CAD build for the part. Positions are in the model's coordinates, mm. A direction names the side the tool comes from. Coordinates: 2 decimals unless noted, no trailing zeros. Write each loop counter-clockwise with the first axis right and the second up, starting at its lowest first coordinate (ties: lowest second). Pieces come first, ordered by that corner, then holes. Notation, with made-up numbers: (39, 25.25) - (93, 25.25) arc R16 cw to (93, 37.25) - close; hole circle Ø8 at (-7.75, 73). An arc over 180 degrees is marked (long way). One line per question, with ' | ' between items. Start each with the question number.
1. Band-saw the part on A-A, the plane x = 0. Write the cut outline in (y, z).
2. Probe line 1 (Z direction, x = -55, y = -20); line 2 (X direction, y = 0, z = -2.25); line 3 (Y direction, x = 0, z = 5.75). List the from-to ranges inside material, lowest first.
3. Two-plate mould, pull along Z, no slides. Class faces 1 (the flat face through (-1, 13, -6.35)), 2 (the flat face through (-1, -13, 12.7)), 3 (the cylindrical face through (-43.06, 39.48, 3.13)), 4 (the flat face through (-10, 58, 6.35)): +Z half, -Z half, draft (parallel to the pull), parting line (faces both ways), or undercut.
4. Band-saw the part on D-D, the plane z = 9.5. Write the cut outline in (x, y), then the cut area to 3 significant figures.
5. Band-saw the part on C-C, the plane x = 23. Write the cut outline in (y, z).
6. Flat gauge pins, fed straight in: P1, Ø8, axis at x = -25, z = 3, coming from the -Y side; P2, Ø3, axis at y = -3.5, z = 2, coming from the -X side; P3, Ø1, axis at y = 2, z = 3, coming from the +X side. Where does each tip first touch, or does it go through?
7. Which spindle directions (+Z, -Z, +X, -X, +Y, -Y) get a long thin tool onto all of the face, cutting with end or side? Do faces 5 (the cylindrical face through (-0.83, 3.72, 3.31)), 6 (the flat face through (-10, -58, 0)). Say none if no direction does.
from build123d import *

# Parameters (mm, degrees)
F0_R     = 58.42
F1_DEPTH = 6.35
F2_R     = 3.81
F3_DEPTH = 25.4
F4_R     = 64.77
F4_R_2   = 58.42
F4_R_3   = 3.81
F5_DEPTH = 6.35
F6_R     = 64.77
F6_R_2   = 58.42
F6_R_3   = 3.81
F7_DEPTH = 6.35


with BuildPart() as f1:
    # F0 (on Top) → F1 (new body)
    with BuildSketch(Plane.XY):
        Circle(F0_R)
    extrude(amount=F1_DEPTH)

    # F2 (on face) → F3 (cut)
    with BuildSketch(Plane.XY.offset(6.35)):
        Circle(F2_R)
    extrude(amount=-F3_DEPTH, mode=Mode.SUBTRACT)

    # F4 (on face) → F5 (join)
    with BuildSketch(Plane.XY.offset(6.35)):
        Circle(F4_R)
        Circle(F4_R_2, mode=Mode.SUBTRACT)
        Circle(F4_R_2)
        Circle(F4_R_3, mode=Mode.SUBTRACT)
    extrude(amount=F5_DEPTH)

    # F6 (on face) → F7 (join)
    with BuildSketch(Plane(origin=(0, 0, 0), x_dir=(1, 0, 0), z_dir=(0, 0, -1))):
        Circle(F6_R)
        Circle(F6_R_2, mode=Mode.SUBTRACT)
        Circle(F6_R_2)
        Circle(F6_R_3, mode=Mode.SUBTRACT)
    extrude(amount=F7_DEPTH)


solid = f1.part
Filled in:
1) outline: (-64.77, -6.35) - (-3.81, -6.35) - (-3.81, 12.7) - (-64.77, 12.7) - (-64.77, 6.35) - (-58.42, 6.35) - (-58.42, 0) - (-64.77, 0) - close; (3.81, -6.35) - (64.77, -6.35) - (64.77, 0) - (58.42, 0) - (58.42, 6.35) - (64.77, 6.35) - (64.77, 12.7) - (3.81, 12.7) - close
2) line 1: z = -6.35 to 0, 6.35 to 12.7 | line 2: x = -64.77 to -3.81, 3.81 to 64.77 | line 3: y = -58.42 to -3.81, 3.81 to 58.42
3) face 1: -Z half | face 2: +Z half | face 3: undercut | face 4: undercut
4) outline: circle Ø129.54 at (0, 0); hole circle Ø7.62 at (0, 0) | area: 13,100 mm²
5) outline: (-60.55, -6.35) - (60.55, -6.35) - (60.55, 0) - (53.7, 0) - (53.7, 6.35) - (60.55, 6.35) - (60.55, 12.7) - (-60.55, 12.7) - (-60.55, 6.35) - (-53.7, 6.35) - (-53.7, 0) - (-60.55, 0) - close
6) P1: stops at y = -60.79 | P2: stops at x = -58.39 | P3: stops at x = 58.4
7) face 5: +Z, -Z | face 6: none
